Here's the drawing with two shaded views (mm, measured from the low corner). I have some questions. A direction names the side the tool comes from. Coordinates: 2 decimals unless noted, no trailing zeros. Loops run counter-clockwise (first coordinate to the right, second up) from the corner with the lowest first, then second, coordinate; pieces in that order, holes last. Notation, with made-up numbers: (9, 42) - (30, 42) arc R28 cw to (30, 73) - close; hole circle Ø7 at (1, 18). An arc over 180 degrees is marked (long way). Use a Markdown table: item, result.
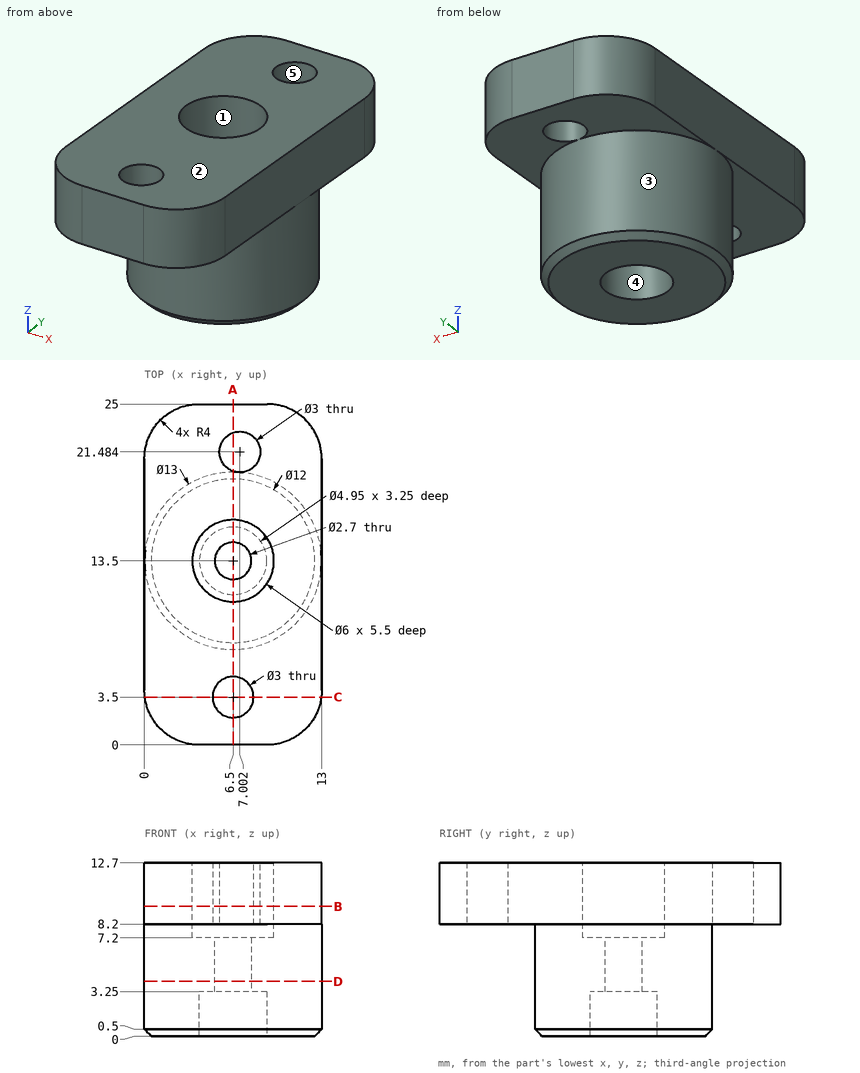
Q1. I want a section at C-C, the plane y = 3.5. Write out the boundary of the cut face in (x, z), then the cut area to 3 significant figures.
Check values:
| item | result |
|---|---|
| outline | (0.03, 8.2) - (5, 8.2) - (5, 12.7) - (0.03, 12.7) - close; (8, 8.2) - (12.97, 8.2) - (12.97, 12.7) - (8, 12.7) - close |
| area | 44.7 mm^2 |
Q2. Will these pins go through, and if not, where does the flat tip stop? P1, Ø3, axis at y = 20.5, z = 6.5, coming from the -X side (1 decimal); P2, Ø2, axis at x = 3, z = 8.5, coming from the -Y side; P3, Ø1.5, axis at x = 11.5, z = 8, coming from the +Y side; P4, Ø1.8, axis at x = 6.5, y = 12, coming from the +Z side.
Check values:
| item | result |
|---|---|
| P1 | x = 3 |
| P2 | y = 0 |
| P3 | y = 24.58 |
| P4 | z = 7.2 |
Q3. Please list where these lines run through material, in increasing order: L1, parallel to Y at x = 6.5, z = 3 (1 decimal); L2, parallel to Z at x = 12.5, y = 22.75; L3, parallel to Y at x = 6.5, z = 9.55. Write a range as from..to.
Check values:
| item | result |
|---|---|
| L1 | 7..11, 16..20 |
| L2 | 8.2..12.7 |
| L3 | 0..2, 5..10.5, 16.5..20.07, 22.9..25 |
Q4. I want a section at B-B, the plane z = 9.5. Write out the boundary of the cut face in (x, y).
Check values:
| item | result |
|---|---|
| outline | (0, 4) arc R4 ccw to (4, 0) - (9, 0) arc R4 ccw to (13, 4) - (13, 21) arc R4 ccw to (9, 25) - (4, 25) arc R4 ccw to (0, 21) - close; hole circle Ø6 at (6.5, 13.5); hole circle Ø3 at (6.5, 3.5); hole circle Ø3 at (7, 21.48) |
Q5. Which directions (+Z, -Z, +X, -X, +Y, -Y) give clear straight access to the entire face, cutting with the end or side of a thin tool? Please do the marked faces 4 and 5.
Check values:
| item | result |
|---|---|
| face 4 | -Z |
| face 5 | +Z, -Z |
Q6. If we mould it in two halves opening along X, with no side actions, what happens to the marked faces 1, 2 and 3? For each: pulls with the +X half, pulls with the -X half, needs draft (parallel to the pull), parting line crosses it, or undercut.
Check values:
| item | result |
|---|---|
| face 1 | undercut |
| face 2 | needs draft |
| face 3 | parting line crosses it |
Q7. I want a section at A-A, the plane x = 6.5. Give the number of separate pieces and of enclosed holes in the cut face, then the cut area to 3 significant figures.
Check values:
| item | result |
|---|---|
| separate pieces | 4 |
| enclosed holes | 0 |
| area | 133 mm^2 |
Q8. I want a section at D-D, the plane z = 4. Write out the boundary of the cut face in (x, y), then the cut area to 3 significant figures.
Check values:
| item | result |
|---|---|
| outline | circle Ø13 at (6.5, 13.5); hole circle Ø2.7 at (6.5, 13.5) |
| area | 127 mm^2 |
